Drawing for the job (mm, zero at the part's lowest x, y, z). A direction names the side the tool comes from. Give positions to 0.01 mm unless a question says otherwise; leave off trailing zeros. Order: outer loops, then holes, each group sorted by start corner. A loop starts at its lowest first (then second) coordinate and runs counter-clockwise, first axis right, second up. Notation, with made-up numbers: (49, 66.5) - (71, 66.5) arc R11 ccw to (71, 81.5) - close; hole circle Ø5 at (54, 22.5). An arc over 180 degrees is marked (long way). One line per item, written item: value.
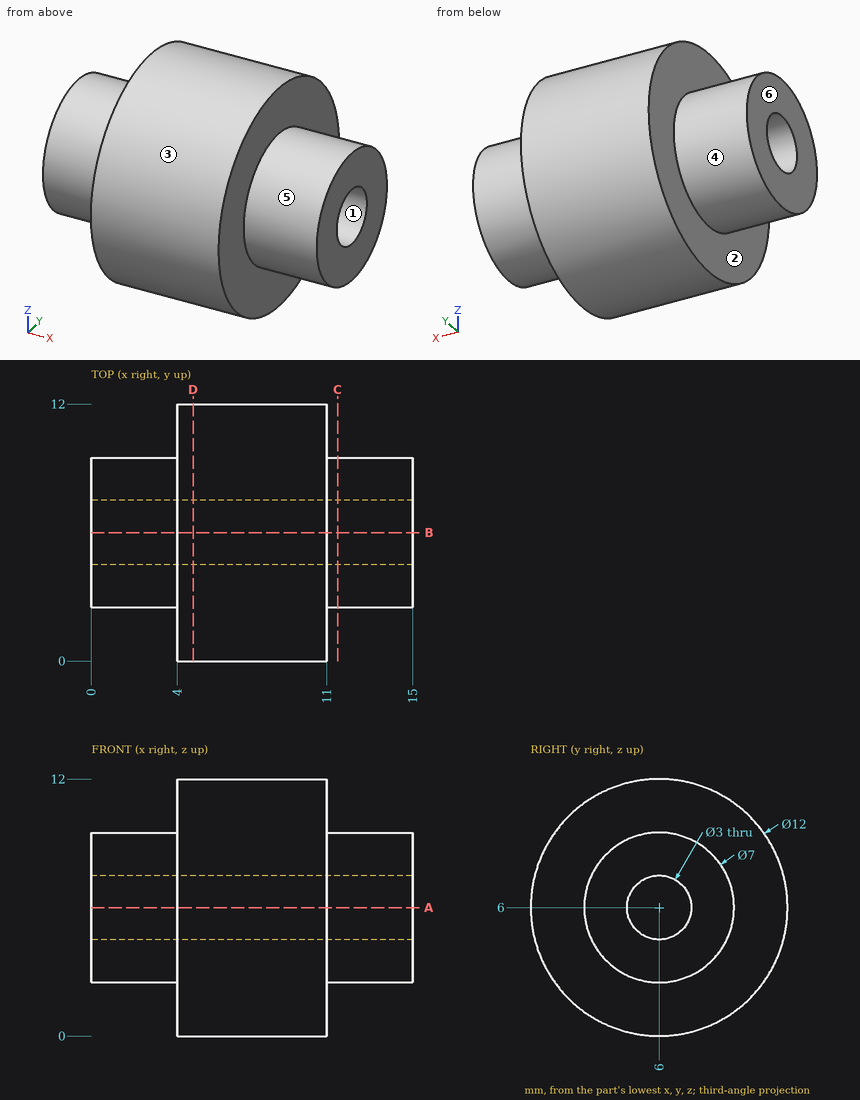
1) Mould opens along Z. For the marked faces 1, 2 and 3 say: released by +Z, released by -Z, zero draft, split by the parting line, or undercut.
Outcome:
face 1: undercut
face 2: zero draft
face 3: split by the parting line
2) Which spindle directions (+Z, -Z, +X, -X, +Y, -Y) get a long thin tool onto all of the face, cutting with end or side? Do the marked faces 4, 5 and 6. Say none if no direction does.
Outcome:
face 4: -X
face 5: +X
face 6: +Z, -Z, -X, +Y, -Y
3) Cut at D-D, the plane x = 4.75. Give the cut face in (y, z), then the cut area to 3 significant figures.
Outcome:
outline: circle Ø12 at (6, 6); hole circle Ø3 at (6, 6)
area: 106 mm^2
4) Cut at C-C, the plane x = 11.5. Give the cut face in (y, z).
Outcome:
outline: circle Ø7 at (6, 6); hole circle Ø3 at (6, 6)
5) Pin check, flat tips, straight feed: pin 1 (1.5 mm diameter, centred on x = 6, z = 3, fed in from +Y); pin 2 (3 mm diameter, centred on x = 10, z = 8, fed in from -Y); pin 3 (2.5 mm diameter, centred on y = 6, z = 6, fed in from -X); pin 4 (5 mm diameter, centred on x = 6, y = 9, fed in from +Z). Stop position of each tip, or through.
Outcome:
pin 1: stops at y = 11.56
pin 2: stops at y = 0.02
pin 3: passes through
pin 4: stops at z = 11.98
6) Drill centre lines: line 1 along X through (y, z) = (10.5, 5.5); line 2 along Z through (x, y) = (1.5, 7.25); line 3 along Z through (x, y) = (10, 2). Where is each one in solid material? Low to high. Write a range as from..to.
Outcome:
line 1: x = 4..11
line 2: z = 2.73..5.17, 6.83..9.27
line 3: z = 1.53..10.47
7) Cut at A-A, the plane z = 6. Give the cut face in (x, y), then the cut area to 3 significant figures.
Outcome:
outline: (0, 2.5) - (4, 2.5) - (4, 0) - (11, 0) - (11, 2.5) - (15, 2.5) - (15, 4.5) - (0, 4.5) - close; (0, 7.5) - (15, 7.5) - (15, 9.5) - (11, 9.5) - (11, 12) - (4, 12) - (4, 9.5) - (0, 9.5) - close
area: 95.0 mm^2
